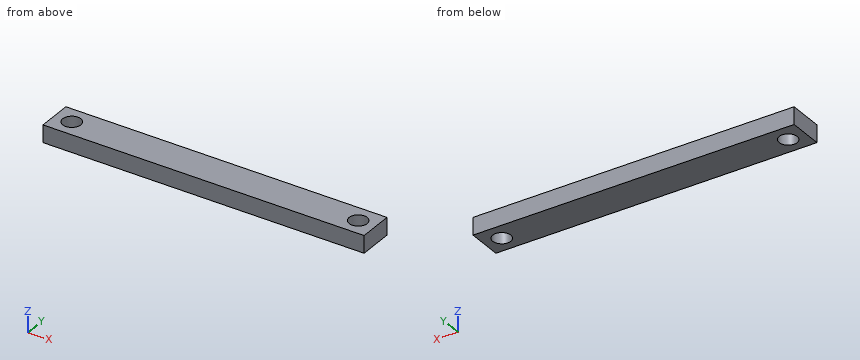
from build123d import *

# Parameters (mm, degrees)
F0_W     = 92.5
F0_H     = 10
F1_DEPTH = 5
F3_DEPTH = 25
F4_R     = 2.6
F5_DEPTH = 25


with BuildPart() as f1:
    # F0 (on Top) → F1 (new body)
    with BuildSketch(Plane.XY):
        Rectangle(F0_W, F0_H)
    extrude(amount=F1_DEPTH)

    # F2 (on face) → F3 (cut)
    with BuildSketch(Plane.XY.offset(5)):
        with BuildLine():
            ThreePointArc((-43.85, 0), (-41.25, -2.6), (-38.65, 0))
            ThreePointArc((-38.65, 0), (-41.25, 2.6), (-43.85, 0))
        make_face()
    extrude(amount=-F3_DEPTH, mode=Mode.SUBTRACT)

    # F4 (on face) → F5 (cut)
    with BuildSketch(Plane.XY.offset(5)):
        with Locations((41.25, 0)):
            Circle(F4_R)
    extrude(amount=-F5_DEPTH, mode=Mode.SUBTRACT)


solid = f1.part
The model under review builds one solid part; all positions refer to its coordinate system, in mm. Coordinates: 2 decimals unless noted, no trailing zeros. Order: outer loops, then holes, each group sorted by start corner. A loop starts at its lowest first (then second) coordinate and runs counter-clockwise, first axis right, second up. Notation, with made-up numbers: (6.5, -9.75) -> (63.5, -9.75) arc R17 ccw to (63.5, 9.25) -> close; hole circle Ø5 at (62, -11). An arc over 180 degrees is marked (long way). Answer in a Markdown table with one row per item.
(1) Consider section B-B (y = 0). Write out the cut boundary in (x, z).
Answers:
| item | result |
|---|---|
| outline | (-46.25, 0) -> (-43.85, 0) -> (-43.85, 5) -> (-46.25, 5) -> close; (-38.65, 0) -> (38.65, 0) -> (38.65, 5) -> (-38.65, 5) -> close; (43.85, 0) -> (46.25, 0) -> (46.25, 5) -> (43.85, 5) -> close |
(2) Wall thickness on line 1 along Y through (x, z) = (41.25, 3.2); line 2 along X through (y, z) = (-0.25, 1.65); line 3 along X through (y, z) = (2.25, 1.55): over which ranges is each line inside the solid? List them lowest first.
Answers:
| item | result |
|---|---|
| line 1 | -5 to -2.6, 2.6 to 5 |
| line 2 | -46.25 to -43.84, -38.66 to 38.66, 43.84 to 46.25 |
| line 3 | -46.25 to -42.55, -39.95 to 39.95, 42.55 to 46.25 |
(3) Consider section A-A (x = 41.25). Write out the cut boundary in (y, z).
Answers:
| item | result |
|---|---|
| outline | (-5, 0) -> (-2.6, 0) -> (-2.6, 5) -> (-5, 5) -> close; (2.6, 0) -> (5, 0) -> (5, 5) -> (2.6, 5) -> close |
(4) Consider section C-C (z = 1.65). Write out the cut boundary in (x, y), plus the area to 3 significant figures.
Answers:
| item | result |
|---|---|
| outline | (-46.25, -5) -> (46.25, -5) -> (46.25, 5) -> (-46.25, 5) -> close; hole circle Ø5.2 at (-41.25, 0); hole circle Ø5.2 at (41.25, 0) |
| area | 883 mm² |
